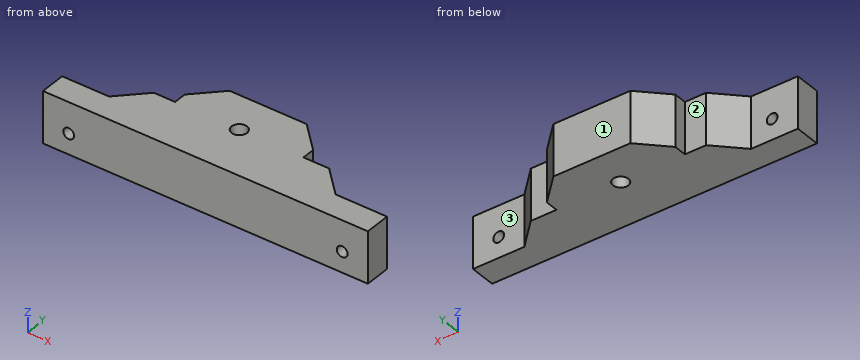
from build123d import *

# Parameters (mm, degrees)
SKETCH_1_W          = 126.5
SKETCH_1_H          = 20
SKETCH_1_R          = 2.1
EXTRUDE_1_DEPTH     = 40
SKETCH_2_R          = 3
CUT_EXTRUDE_1_DEPTH = 322.481529503
CHAMFER_1_SIZE      = 10
CHAMFER_2_SIZE      = 10


with BuildPart() as part:
    # Эскиз1 → Бобышка-Вытянуть1 (new body)
    with BuildSketch(Plane(origin=(0, 254.195974268, 0), x_dir=(1, 0, 0), z_dir=(0, 1, 0))):
        with Locations((64.808980694, -42.273129836)):
            Rectangle(SKETCH_1_W, SKETCH_1_H)
        with Locations(Location((11.55898069, -40.273129836, 0), (0, 0, 180))):
            Circle(SKETCH_1_R, mode=Mode.SUBTRACT)
        with Locations(Location((118.058980694, -40.273129836, 0), (0, 0, 180))):
            Circle(SKETCH_1_R, mode=Mode.SUBTRACT)
    extrude(amount=EXTRUDE_1_DEPTH)

    # Эскиз2 → Вырез-Вытянуть1 (cut, through all)
    with BuildSketch(Plane(origin=(0, 0, 32.273129836), x_dir=(-1, 0, 0), z_dir=(0, 0, -1))):
        with Locations(Location((-63.058980694, 274.145974268, 0), (0, 0, 90))):
            Circle(SKETCH_2_R)
        Polygon((-128.058980694, 294.195974268), (-128.058980694, 274.195974268), (-128.058980694, 264.145974268), (-108.058980694, 264.145974268), (-108.058980694, 274.145974268), (-88.058980694, 274.145974268), (-88.058980694, 289.145974268), (-38.058980694, 289.145974268), (-38.058980694, 274.145974268), (-19.808980694, 274.145974268), (-19.808980694, 264.145974268), (-1.558980694, 264.145974268), (-1.558980694, 274.195974268), (-1.558980694, 294.195974268), align=None)
    extrude(amount=-CUT_EXTRUDE_1_DEPTH, mode=Mode.SUBTRACT)

    # Фаска1
    chamfer_1_edges = [part.edges().sort_by_distance(p)[0] for p in [
        (38.058980694, 289.145974268, 42.273129836),
        (88.058980694, 289.145974268, 42.273129836),
    ]]
    chamfer(chamfer_1_edges, length=CHAMFER_1_SIZE)

    # Фаска2
    chamfer_2_edges = [part.edges().sort_by_distance(p)[0] for p in [
        (19.808980694, 274.145974268, 42.273129836),
        (108.058980694, 274.145974268, 42.273129836),
    ]]
    chamfer(chamfer_2_edges, length=CHAMFER_2_SIZE - 0.0001)  # a hair under: the kernel refuses the full size


solid = part.part
Read the model definition and answer for the solid it produces. Units are mm, in the model's axes. Face numbers are marked on the shaded views. A direction names the side the tool comes from. Coordinates: 2 decimals unless noted, no trailing zeros. Order: outer loops, then holes, each group sorted by start corner. A loop starts at its lowest first (then second) coordinate and runs counter-clockwise, first axis right, second up. Notation, with made-up numbers: M 4.25,70.25 L 55.25,70.25 A30 cw 55.25,95.25 Z; hole C 37.5,-15 d11. An arc over 180 degrees is marked long. Put each result on its own line as item: value. Start each with the question number.
Item 1: Consider probe 1 along Y at (x, z) = (18.5, 44.25); probe 2 along X at (y, z) = (273.5, 48.25); probe 3 along Y at (x, z) = (90, 50). Determine where each line is inside the solid, lowest interval first. Write a range as [from, to].
Item 2: For the marked faces 1, 2 and 3, determine the directions among +Z, -Z, +X, -X, +Y, -Y from which every point of the face is accessible in a straight line to the end or side of a thin tool.
Item 3: Given pin 1 Ø10 at (x, y) = (87.5, 281) entering from -Z; pin 2 Ø2.5 at (x, z) = (35.5, 42) entering from +Y; pin 3 Ø1.5 at (y, z) = (276.5, 37.5) entering from -X; pin 4 Ø6 at (x, z) = (121.5, 39) entering from +Y, each flat-ended and moving along its own axis, determine where each tip first touches the part or whether it passes through.
Item 4: Section D-D, the plane x = 31.5 is taken. Determine the outline of the cut face in (y, z), plus the area to 3 significant figures.
Item 5: Section A-A, the plane x = 117.5 is taken. Determine the outline of the cut face in (y, z).
Item 6: Section B-B, the plane y = 275.5 is taken. Determine the outline of the cut face in (x, z).
Computed:
1. probe 1: y = [254.2, 264.15]
1. probe 2: x = [29.16, 60.13], [65.99, 98.71]
1. probe 3: y = [254.2, 274.15]
2. face 1: +Z, -Z, +X, -X, +Y
2. face 2: +Z, -Z, -X, +Y
2. face 3: +Z, -Z, +X, +Y
3. pin 1: stops at z = 32.27
3. pin 2: stops at y = 274.15
3. pin 3: stops at x = 38.06
3. pin 4: stops at y = 264.15
4. outline: M 254.2,32.27 L 274.15,32.27 L 274.15,52.27 L 254.2,52.27 Z
4. area: 399 mm2
5. outline: M 254.2,32.27 L 264.15,32.27 L 264.15,38.25 L 254.2,38.25 Z; M 254.2,42.3 L 264.15,42.3 L 264.15,52.27 L 254.2,52.27 Z
6. outline: M 38.06,32.27 L 60.38,32.27 L 60.38,52.27 L 38.06,52.27 Z; M 65.74,32.27 L 88.06,32.27 L 88.06,52.27 L 65.74,52.27 Z
